Model file for the job. Use its own axes, mm. A direction names the side the tool comes from. Round coordinates to 2 decimals unless told otherwise and drop trailing zeros. Write each loop counter-clockwise with the first axis right and the second up, starting at its lowest first coordinate (ties: lowest second). Pieces come first, ordered by that corner, then holes.
Autodesk Inventor part; units mm, degrees
ref_plane "YZ Plane" through (0, 0, 0) normal (1, 0, 0) x (0, 1, 0)
ref_plane "XZ Plane" through (0, 0, 0) normal (0, 1, 0) x (-1, 0, 0)
ref_plane "XY Plane" through (0, 0, 0) normal (0, 0, 1) x (1, 0, 0)
sketch "Sketch1" plane through (0, 0, 0) normal (0, 0, 1) x (1, 0, 0)
  line L0 (4.25, 1.75) -> (-4.25, 1.75)
  line L1 (-4.25, 1.75) -> (-4.25, -1.75)
  line L2 (-4.25, -1.75) -> (4.25, -1.75)
  line L3 (4.25, -1.75) -> (4.25, 1.75)
  line L4 (4.25, 1.75) -> (-4.25, -1.75) construction
  line L5 (-4.25, 1.75) -> (4.25, -1.75) construction
  point P0 (0, 0)
  dimension "d0" = 8.5
  dimension "d1" = 3.5
extrude "Extrusion1" add sketch "Sketch1" along normal blind 3.5
sketch "Sketch2" plane through (0, 0, 3.5) normal (0, 0, 1) x (1, 0, 0)
  line L0 (1.8, 0.82) -> (-1.8, 0.82)
  line L1 (-1.8, 0.82) -> (-1.8, -0.82)
  line L2 (-1.8, -0.82) -> (1.8, -0.82)
  line L3 (1.8, -0.82) -> (1.8, 0.82)
  line L4 (1.8, 0.82) -> (-1.8, -0.82) construction
  line L5 (-1.8, 0.82) -> (1.8, -0.82) construction
  point P0 (0, 0)
  dimension "d4" = 3.6
  dimension "d5" = 1.64
extrude "Extrusion2" cut sketch "Sketch2" against normal blind 1
sketch "Sketch3" plane through (0, 0, 2.5) normal (0, 0, 1) x (1, 0, 0)
  line L0 (-1.8, -0.82) -> (-1.8, 0.82)
  line L1 (1.8, -0.82) -> (-1.8, -0.82)
  line L2 (1.8, 0.82) -> (1.8, -0.82)
  line L3 (-1.8, 0.82) -> (1.8, 0.82)
  line L4 (1.8, 0.82) -> (0.16, 0.82)
  line L5 (0.16, 0.82) -> (0.16, -0.82)
  line L6 (0.16, -0.82) -> (1.8, -0.82)
  line L7 (1.8, -0.82) -> (1.8, 0.82)
  point P0 (0, 0)
  dimension "d8" = 1.64
extrude "Extrusion3" add sketch "Sketch3" along normal blind 4 contours L5 L3 L2 L1
fillet "Fillet1" radius 0.5 4 edges at (0, 1.75, 3.5) (-4.25, 0, 3.5) (0, -1.75, 3.5) (4.25, 0, 3.5)
chamfer "Chamfer1" distance 0.2 angle 45 4 edges at (0.98, 0.82, 6.5) (0.16, 0, 6.5) (0.98, -0.82, 6.5) (1.8, 0, 6.5)
sketch "Sketch4" plane through (0, 0, 0) normal (0, 0, -1) x (-1, 0, 0)
  line L0 (-2.75, 0.15) -> (-2.25, 0.15)
  line L1 (-2.25, 0.15) -> (-2.25, -0.15)
  line L2 (-2.25, -0.15) -> (-2.75, -0.15)
  line L3 (-2.75, -0.15) -> (-2.75, 0.15)
  line L4 (-0.25, 0.15) -> (0.25, 0.15)
  line L5 (0.25, 0.15) -> (0.25, -0.15)
  line L6 (0.25, -0.15) -> (-0.25, -0.15)
  line L7 (-0.25, -0.15) -> (-0.25, 0.15)
  line L8 (2.25, 0.15) -> (2.75, 0.15)
  line L9 (2.75, 0.15) -> (2.75, -0.15)
  line L10 (2.75, -0.15) -> (2.25, -0.15)
  line L11 (2.25, -0.15) -> (2.25, 0.15)
  point P0 (0, 0)
  point P1 (0, 0.15)
  point P2 (-2.5, 0.15)
  point P3 (2.5, 0.15)
  dimension "d15" = 0.5
  dimension "d16" = 0.3
  dimension "d17" = 0.5
  dimension "d18" = 0.3
  dimension "d19" = 0.5
  dimension "d20" = 0.3
  dimension "d21" = 2.5
  dimension "d22" = 2.5
  dimension "d24" = 0.15
  dimension "d25" = 0.25
extrude "Extrusion4" add sketch "Sketch4" along normal blind 3.7
properties part number "switch"
1) Cut at D-D on z = 4.75. List the corners of the cut face in (x, y).
2) Cut at A-A on z = -1.25. List the corners of the cut face in (x, y).
3) Wall check: probe 1 along Z at (x, y) = (-2.25, -0.6); probe 2 along Z at (x, y) = (-0.5, -0.4); probe 3 along X at (y, z) = (0.2, 4.25). Give the ranges that are in metal, low to high.
4) Pull direction Y, two halves, no side cores. Call faces 1 (the face through (-1, 0.82, 3)), 2 (the face through (-1.8, 0, 3)), 3 (the face through (1, -0.82, 5)), 4 (the face through (0, 1, 3.5)): released by +Y, released by -Y, zero draft, split by the parting line, or undercut.
5) Cut at B-B on x = -1. List the corners of the cut face in (y, z).
6) Which spindle directions (+Z, -Z, +X, -X, +Y, -Y) get a long thin tool onto all of the face, cutting with end or side? Do faces 5 (the face through (1.8, 0, 5)), 6 (the face through (4.25, 0, 1)), 7 (the face through (1, 0, 6.5)), 8 (the face through (-1, -0.82, 3)), 9 (the face through (1, 0.82, 5)). Say none if no direction does.
7) Cut at C-C on x = 3.5. List the corners of the cut face in (y, z), and give its area (3 significant figures).
8) Flat gauge pins, fed straight in: pin 1 Ø0.8 at (x, z) = (1, 5) entering from -Y; pin 2 Ø1.8 at (y, z) = (0, 4.5) entering from +X; pin 3 Ø0.6 at (x, z) = (2.5, -1) entering from -Y. Where does each tip first touch, or does it go through?
Result sheet:
1. outline: (0.16, -0.82) - (1.8, -0.82) - (1.8, 0.82) - (0.16, 0.82) - close
2. outline: (-2.75, -0.15) - (-2.25, -0.15) - (-2.25, 0.15) - (-2.75, 0.15) - close; (-0.25, -0.15) - (0.25, -0.15) - (0.25, 0.15) - (-0.25, 0.15) - close; (2.25, -0.15) - (2.75, -0.15) - (2.75, 0.15) - (2.25, 0.15) - close
3. probe 1: z = 0 to 3.5
3. probe 2: z = 0 to 2.5
3. probe 3: x = 0.16 to 1.8
4. face 1: undercut
4. face 2: undercut
4. face 3: released by -Y
4. face 4: zero draft
5. outline: (-1.75, 0) - (1.75, 0) - (1.75, 3) arc R0.5 ccw to (1.25, 3.5) - (0.82, 3.5) - (0.82, 2.5) - (-0.82, 2.5) - (-0.82, 3.5) - (-1.25, 3.5) arc R0.5 ccw to (-1.75, 3) - close
6. face 5: +Z, +X, +Y, -Y
6. face 6: +Z, -Z, +X, +Y, -Y
6. face 7: +Z, +X, -X, +Y, -Y
6. face 8: +Z
6. face 9: +Z, +X, -X, +Y
7. outline: (-1.75, 0) - (1.75, 0) - (1.75, 3) arc R0.5 ccw to (1.25, 3.5) - (-1.25, 3.5) arc R0.5 ccw to (-1.75, 3) - close
7. area: 12.1 mm2
8. pin 1: stops at y = -0.82
8. pin 2: stops at x = 1.8
8. pin 3: stops at y = -0.15
